Source: three-view drawing plus pictorial views. Frame: mm from the lowest corner of the part. A direction names the side the tool comes from. Round coordinates to 2 decimals unless told otherwise and drop trailing zeros. Loops run counter-clockwise (first coordinate to the right, second up) from the corner with the lowest first, then second, coordinate; pieces in that order, holes last. Notation, with made-up numbers: (30, 37.5) -> (43, 37.5) arc R30 ccw to (43, 59.5) -> close; hole circle Ø2 at (-8.5, 36). An arc over 180 degrees is marked (long way). Answer in a Markdown table with one row per item.
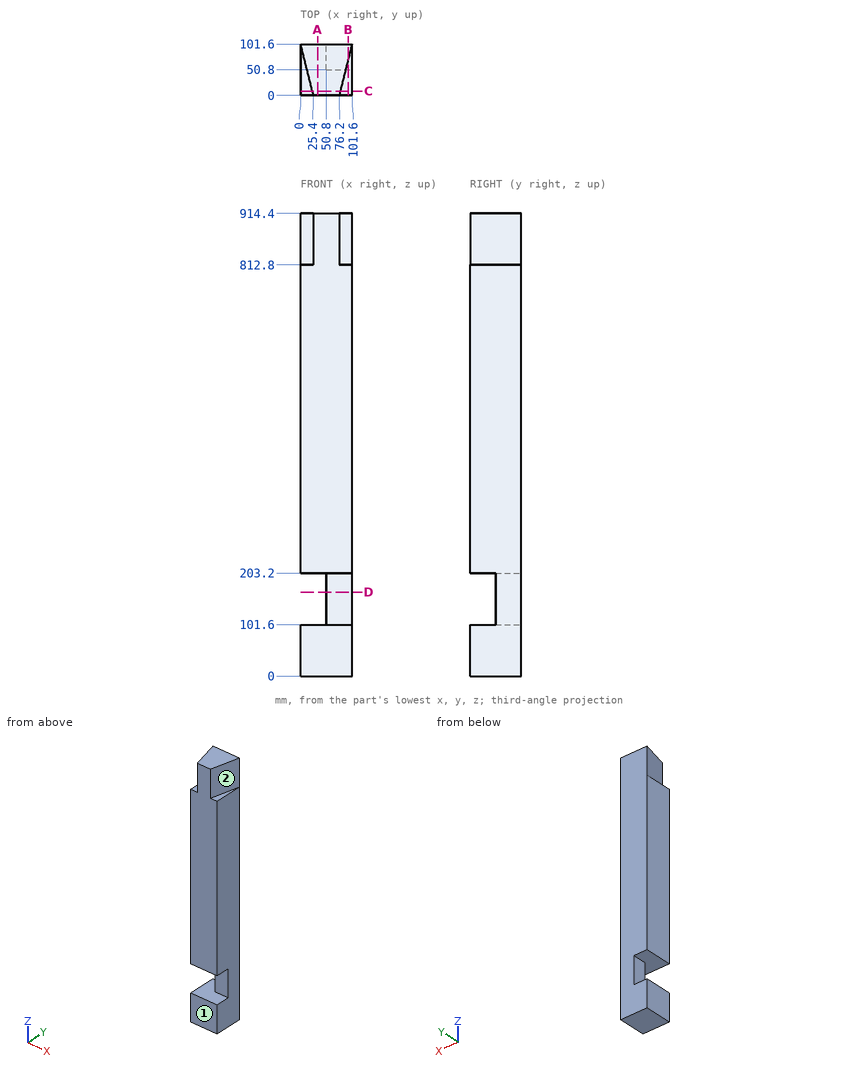
Item 1: Reachability of the marked faces 1 and 2 from +Z, -Z, +X, -X, +Y, -Y: full face, straight path, thin tool, end or side. Return the list, or none.
Answer:
| item | result |
|---|---|
| face 1 | +Z, -Z, +X, -X, -Y |
| face 2 | +Z, +X, -Y |
Item 2: Cut plane C-C (y = 8.5). Output: boundary loops of the cut face in (x, z) (3 decimals), then the cut area to 3 significant figures.
Answer:
| item | result |
|---|---|
| outline | (0, 0) -> (101.6, 0) -> (101.6, 101.6) -> (0, 101.6) -> close; (0, 203.2) -> (101.6, 203.2) -> (101.6, 812.8) -> (78.325, 812.8) -> (78.325, 914.4) -> (23.275, 914.4) -> (23.275, 812.8) -> (0, 812.8) -> close |
| area | 77,900 mm² |
Item 3: Cut plane B-B (x = 94). Output: boundary loops of the cut face in (y, z).
Answer:
| item | result |
|---|---|
| outline | (0, 0) -> (101.6, 0) -> (101.6, 914.4) -> (71.2, 914.4) -> (71.2, 812.8) -> (0, 812.8) -> (0, 203.2) -> (50.8, 203.2) -> (50.8, 101.6) -> (0, 101.6) -> close |
Item 4: Pin query (flat end, axial travel): pin 1 Ø15 at (x, z) = (87, 132) entering from -Y. Return the tip coordinate at first contact, or that it passes through.
Answer:
| item | result |
|---|---|
| pin 1 | stops at y = 50.8 |
Item 5: Cut plane D-D (z = 166). Output: boundary loops of the cut face in (x, y).
Answer:
| item | result |
|---|---|
| outline | (50.8, 50.8) -> (101.6, 50.8) -> (101.6, 101.6) -> (50.8, 101.6) -> close |
Item 6: Line query: probe 1 along Z at (x, y) = (80.5, 34.5); probe 2 along Z at (x, y) = (87, 42); probe 3 along X at (y, z) = (58.5, 177). Output: solid intervals per line, ascending. Write a range as [from, to].
Answer:
| item | result |
|---|---|
| probe 1 | z = [0, 101.6], [203.2, 914.4] |
| probe 2 | z = [0, 101.6], [203.2, 812.8] |
| probe 3 | x = [50.8, 101.6] |
Item 7: Cut plane A-A (x = 33.5). Output: boundary loops of the cut face in (y, z), then the cut area to 3 significant figures.
Answer:
| item | result |
|---|---|
| outline | (0, 0) -> (101.6, 0) -> (101.6, 101.6) -> (0, 101.6) -> close; (0, 203.2) -> (101.6, 203.2) -> (101.6, 914.4) -> (0, 914.4) -> close |
| area | 82,600 mm² |
